from build123d import *

# Parameters (mm, degrees)
CROQUIS1_R              = 1.1
CROQUIS1_R_2            = 0.8
CROQUIS1_W              = 40
CROQUIS1_H              = 19
SALIENTE_EXTRUIR1_DEPTH = 8
CROQUIS3_W              = 7
CROQUIS3_H              = 1.8
CORTAR_EXTRUIR2_DEPTH   = 0.8
CROQUIS2_R              = 10
CORTAR_EXTRUIR4_DEPTH   = 129.798291914


with BuildPart() as part:
    # Croquis1 → Saliente-Extruir1 (new body)
    with BuildSketch(Plane(origin=(0, 0, 0), x_dir=(1, 0, 0), z_dir=(0, 1, 0))):
        with BuildLine():
            Line((1.5, 29.962476533), (101.25, 24.968730444))
            ThreePointArc((101.25, 24.968730444), (125, 0), (101.25, -24.968730444))
            Line((101.25, -24.968730444), (1.5, -29.962476533))
            ThreePointArc((1.5, -29.962476533), (-30, 0), (1.5, 29.962476533))
        make_face()
        with Locations(Location((110.89, 5, 0), (0, 0, 270))):
            Circle(CROQUIS1_R, mode=Mode.SUBTRACT)
        with Locations(Location((110.89, -5, 0), (0, 0, 270))):
            Circle(CROQUIS1_R, mode=Mode.SUBTRACT)
        with Locations(Location((61.111607097, -5.4, 0), (0, 0, 270))):
            Circle(CROQUIS1_R, mode=Mode.SUBTRACT)
        with Locations(Location((61.111607097, 4.6, 0), (0, 0, 270))):
            Circle(CROQUIS1_R, mode=Mode.SUBTRACT)
        with Locations(Location((7.5, 0, 0), (0, 0, 270))):
            Circle(CROQUIS1_R_2, mode=Mode.SUBTRACT)
        with Locations(Location((0, -7.5, 0), (0, 0, 270))):
            Circle(CROQUIS1_R_2, mode=Mode.SUBTRACT)
        with Locations(Location((-7.5, 0, 0), (0, 0, 270))):
            Circle(CROQUIS1_R_2, mode=Mode.SUBTRACT)
        with Locations(Location((0, 7.5, 0), (0, 0, 270))):
            Circle(CROQUIS1_R_2, mode=Mode.SUBTRACT)
        with Locations(Location((0, 0, 0), (0, 0, 270))):
            Circle(CROQUIS1_R_2, mode=Mode.SUBTRACT)
        with Locations((86, 0)):
            Rectangle(CROQUIS1_W, CROQUIS1_H, mode=Mode.SUBTRACT)
    extrude(amount=SALIENTE_EXTRUIR1_DEPTH)

    # Croquis3 → Cortar-Extruir2 (cut)
    with BuildSketch(Plane.XZ):
        with Locations((62.5, 0.4)):
            Rectangle(CROQUIS3_W, CROQUIS3_H)
        with Locations((109.5, 0.4)):
            Rectangle(CROQUIS3_W, CROQUIS3_H)
    extrude(amount=-CORTAR_EXTRUIR2_DEPTH, mode=Mode.SUBTRACT)

    # Croquis2 → Cortar-Extruir4 (cut, through all)
    with BuildSketch(Plane.XZ):
        with Locations(Location((0, 0, 0), (0, 0, 270))):
            Circle(CROQUIS2_R)
    extrude(amount=-CORTAR_EXTRUIR4_DEPTH, mode=Mode.SUBTRACT)


solid = part.part
Read the model definition and answer for the solid it produces. Units are mm, in the model's axes. A direction names the side the tool comes from. Give positions to 0.01 mm unless a question says otherwise; leave off trailing zeros. Write each loop counter-clockwise with the first axis right and the second up, starting at its lowest first coordinate (ties: lowest second). Pieces come first, ordered by that corner, then holes. Notation, with made-up numbers: (63, 19.25) - (78, 19.25) arc R14 ccw to (78, 32.25) - close; hole circle Ø5 at (24, -27). An arc over 180 degrees is marked (long way). Use CSV: the item, a comma, the result in double quotes. Start each with the question number.
Item 1: The part is cut by section D-D, the plane x = 44.5. Give the vertices of the cut face in (y, z), and give its area (3 significant figures).
Item 2: The part is cut by section A-A, the plane x = 0. Give the vertices of the cut face in (y, z), and give its area (3 significant figures).
Item 3: The mould has two halves that part along Z. Classify faces 1 (the cylindrical face through (124.994, 3.944, -0.532)), 2 (the flat face through (52.07, 3.94, 27.43)), 3 (the flat face through (86, 4, -9.5)): pulls with the +Z half, pulls with the -Z half, needs draft (parallel to the pull), parting line crosses it, or undercut.
Item 4: For faces 4 (the flat face through (66, 4, 0)), 5 (the flat face through (50.7, 3.9, -27.5)), determine the directions among +Z, -Z, +X, -X, +Y, -Y from which every point of the face is accessible in a straight line to the end or side of a thin tool.
Item 5: The part is cut by section B-B, the plane y = 2.25. Give the vertices of the cut face in (x, z), and give its area (3 significant figures).
Item 6: Flat-ended cylindrical pins translate along their axes: P1, Ø0.6, axis at x = 110.5, y = 0.5, coming from the +Z side; P2, Ø2.5, axis at x = 80, y = 4, coming from the -Z side; P3, Ø4, axis at y = 6.5, z = -16.5, coming from the -X side; P4, Ø2, axis at x = 110.89, z = 5, coming from the +Y side. Find the tip coordinate at first contact, or state that the pin passes through.
Item 7: The part is cut by section C-C, the plane z = 18. Give the vertices of the cut face in (x, y).
Item 8: Consider line 1 (X direction, y = 5.5, z = -6.5); line 2 (Z direction, x = 110.89, y = 5.5); line 3 (X direction, y = 5, z = -5). Determine where each line is inside the solid, lowest interval first.
Taken from the geometry:
1,outline,"(0, -27.81) - (8, -27.81) - (8, 27.81) - (0, 27.81) - close"
1,area,"445 mm2"
2,outline,"(0, -30) - (8, -30) - (8, -10) - (0, -10) - close; (0, 10) - (8, 10) - (8, 30) - (0, 30) - close"
2,area,"320 mm2"
3,face 1,"parting line crosses it"
3,face 2,"pulls with the +Z half"
3,face 3,"undercut"
4,face 4,"+Y, -Y"
4,face 5,"-Z, +X, +Y, -Y"
5,outline,"(1.5, -29.96) - (101.25, -24.97) arc R25 ccw to (101.25, 24.97) - (1.5, 29.96) arc R30 ccw (long way) to start; hole circle Ø20 at (0, 0); hole circle Ø2.2 at (61.11, -4.6); hole circle Ø2.2 at (61.11, 5.4); hole (66, -9.5) - (106, -9.5) - (106, 9.5) - (66, 9.5) - close; hole circle Ø2.2 at (110.89, -5); hole circle Ø2.2 at (110.89, 5)"
5,area,"6,810 mm2"
6,P1,"z = 22.82"
6,P2,"z = -26.1"
6,P3,"x = -26.26"
6,P4,"through"
7,outline,"(-24, 0) - (117.35, 0) - (117.35, 8) - (-24, 8) - close"
8,line 1,"-29.29 to -7.6, 7.6 to 66, 106 to 124.14"
8,line 2,"-22.5 to -6.1, -3.9 to 3.9, 6.1 to 22.5"
8,line 3,"-29.58 to -8.66, 8.66 to 60.09, 62.14 to 66, 106 to 109.79, 111.99 to 124.49"
